Build history of the part. All positions in model axes, mm. Face numbers are marked on the shaded views. A direction names the side the tool comes from. Give positions to 0.01 mm unless a question says otherwise; leave off trailing zeros. Loops run counter-clockwise (first coordinate to the right, second up) from the corner with the lowest first, then second, coordinate; pieces in that order, holes last.
1) Band-saw the part on D-D on z = 17. List the corners of the cut face in (x, y), then the cut area to 3 significant figures.
2) Two-plate mould, pull along Z, no slides. Class the marked faces 1, 2 and 3: +Z half, -Z half, draft (parallel to the pull), parting line (faces both ways), or undercut.
3) Flat gauge pins, fed straight in: P1, Ø1.5, axis at x = -20.33, z = -8.42, coming from the +Y side; P2, Ø3.5, axis at x = 0, z = -19.5, coming from the +Y side; P3, Ø4, axis at x = 16, y = 12.5, coming from the +Z side. Where does each tip first touch, or does it go through?
4) Band-saw the part on B-B on z = 0. List the corners of the cut face in (x, y).
5) Band-saw the part on A-A on x = 0. List the corners of the cut face in (y, z).
6) Wall check: line 1 (Y direction, x = -16, z = 22); line 2 (X direction, y = 18.5, z = 0); line 3 (X direction, y = 22.25, z = 9). Give the ranges that are in metal, low to high.
7) Band-saw the part on C-C on y = 4.75. List the corners of the cut face in (x, z), then the cut area to 3 significant figures.
8) 3-axis set-ups, long thin cutter, end or side, ignore diameter. For the marked faces 4 and 5: which of +Z, -Z, +X, -X, +Y, -Y reach the whole face in a straight line?
```python
from build123d import *

# Parameters (mm, degrees)
ESQUISSE1_W                                   = 50
ESQUISSE1_H                                   = 50
BOSS_EXTRU_1_DEPTH                            = 25
TROU_POUR_TARAUDAGE_POUR_TROU_TARAUD_M3_D     = 2.5
TROU_POUR_TARAUDAGE_POUR_TROU_TARAUD_M3_DEPTH = 10
TROU_POUR_TARAUDAGE_POUR_TROU_TARAUD_M3_TIP   = 0.751075774
TROU_POUR_TARAUDAGE_POUR_TROU_TARAUD_M6_D     = 5
TROU_POUR_TARAUDAGE_POUR_TROU_TARAUD_M6_DEPTH = 10
TROU_POUR_TARAUDAGE_POUR_TROU_TARAUD_M6_TIP   = 1.502151548
ESQUISSE12_W                                  = 4.07874476
ESQUISSE12_H                                  = 14
ENL_V_MAT_EXTRU_1_DEPTH                       = 2
CHANFREIN1_SIZE                               = 1.5


with BuildPart() as part:
    # Esquisse1 → Boss.-Extru.1 (new body)
    with BuildSketch(Plane(origin=(0, 0, 0), x_dir=(1, 0, 0), z_dir=(0, 1, 0))):
        Rectangle(ESQUISSE1_W, ESQUISSE1_H)
    extrude(amount=BOSS_EXTRU_1_DEPTH)

    # Esquisse2 → Enlèvement de matière-Révolution1 (revolve, cut)
    with BuildSketch(Plane.XY, mode=Mode.PRIVATE) as enl_vement_de_mati_re_r_volution1_sk:
        Polygon((0, 0), (4.5, 0), (4.5, 7), (12.5, 15), (12.5, 25), (0, 25), align=None)
    revolve(enl_vement_de_mati_re_r_volution1_sk.sketch.rotate(Axis((0, 0, 0), (0, 1, 0)), 90), axis=Axis((0, 0, 0), (0, 1, 0)), mode=Mode.SUBTRACT)

    # Trou pour taraudage pour trou taraudé M31
    with Locations(Plane(origin=(0, 25, 0), x_dir=(1, 0, 0), z_dir=(0, 1, 0))):
        with Locations((-8.419035512, 20.325349715), (8.419035512, 20.325349715), (20.325349715, 8.419035512), (20.325349715, -8.419035512), (8.419035512, -20.325349715), (-8.419035512, -20.325349715), (-20.325349715, -8.419035512), (-20.325349715, 8.419035512)):
            Hole(TROU_POUR_TARAUDAGE_POUR_TROU_TARAUD_M3_D / 2, depth=TROU_POUR_TARAUDAGE_POUR_TROU_TARAUD_M3_DEPTH)
            with Locations((0, 0, -(TROU_POUR_TARAUDAGE_POUR_TROU_TARAUD_M3_DEPTH + TROU_POUR_TARAUDAGE_POUR_TROU_TARAUD_M3_TIP / 2))):  # 118° drill point
                Cone(0, TROU_POUR_TARAUDAGE_POUR_TROU_TARAUD_M3_D / 2, TROU_POUR_TARAUDAGE_POUR_TROU_TARAUD_M3_TIP, mode=Mode.SUBTRACT)

    # Trou pour taraudage pour trou taraudé M61
    with Locations(Plane.XY.offset(25)):
        with Locations((-16, 12.5), (16, 12.5)):
            Hole(TROU_POUR_TARAUDAGE_POUR_TROU_TARAUD_M6_D / 2, depth=TROU_POUR_TARAUDAGE_POUR_TROU_TARAUD_M6_DEPTH)
            with Locations((0, 0, -(TROU_POUR_TARAUDAGE_POUR_TROU_TARAUD_M6_DEPTH + TROU_POUR_TARAUDAGE_POUR_TROU_TARAUD_M6_TIP / 2))):  # 118° drill point
                Cone(0, TROU_POUR_TARAUDAGE_POUR_TROU_TARAUD_M6_D / 2, TROU_POUR_TARAUDAGE_POUR_TROU_TARAUD_M6_TIP, mode=Mode.SUBTRACT)

    # Esquisse12 → Enlèv. mat.-Extru.1 (cut)
    with BuildSketch(Plane(origin=(0, 25, 0), x_dir=(1, 0, 0), z_dir=(0, 1, 0))):
        with Locations((0, 18)):
            Rectangle(ESQUISSE12_W, ESQUISSE12_H)
    extrude(amount=-ENL_V_MAT_EXTRU_1_DEPTH, mode=Mode.SUBTRACT)

    # Chanfrein1
    chanfrein1_edges = [part.edges().sort_by_distance(p)[0] for p in [
        (0, 25, 12.5),
    ]]
    chamfer(chanfrein1_edges, length=CHANFREIN1_SIZE)


solid = part.part
```
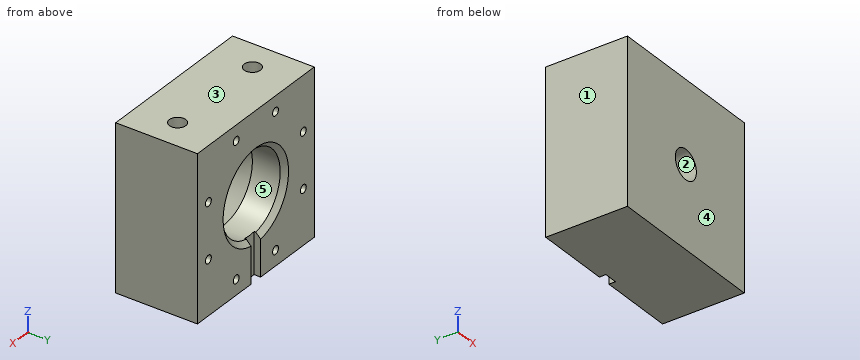
Findings below:
1. outline: (-25, 0) - (25, 0) - (25, 25) - (-25, 25) - close; hole circle Ø5 at (-16, 12.5); hole circle Ø5 at (16, 12.5)
1. area: 1,210 mm2
2. face 1: draft
2. face 2: undercut
2. face 3: +Z half
3. P1: stops at y = 14.7
3. P2: stops at y = 23
3. P3: stops at z = 14.7
4. outline: (-25, 0) - (-4.5, 0) - (-4.5, 7) - (-12.5, 15) - (-12.5, 23.5) - (-14, 25) - (-25, 25) - close; (4.5, 0) - (25, 0) - (25, 25) - (14, 25) - (12.5, 23.5) - (12.5, 15) - (4.5, 7) - close
5. outline: (0, -25) - (23, -25) - (23, -12.5) - (15, -12.5) - (7, -4.5) - (0, -4.5) - close; (0, 4.5) - (7, 4.5) - (15, 12.5) - (23.5, 12.5) - (25, 14) - (25, 25) - (0, 25) - close
6. line 1: y = 0 to 10, 15 to 25
6. line 2: x = -25 to -12.5, 12.5 to 25
6. line 3: x = -25 to -21.43, -19.22 to -8.67, 8.67 to 19.22, 21.43 to 25
7. outline: (-25, -25) - (25, -25) - (25, 25) - (-25, 25) - close; hole circle Ø9 at (0, 0)
7. area: 2,440 mm2
8. face 4: +Z, -Z, +X, -X, -Y
8. face 5: +Y
